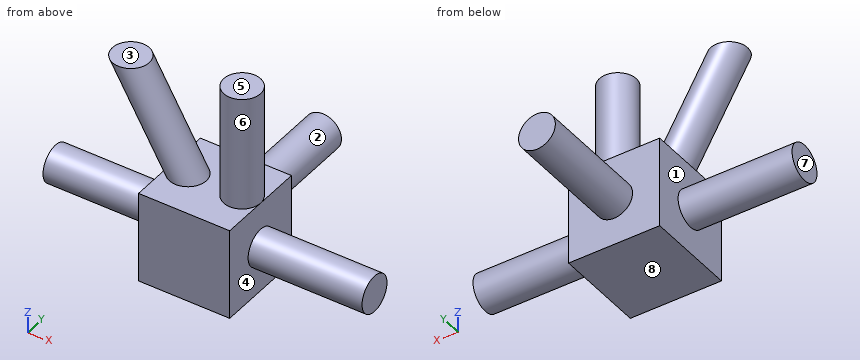
from build123d import *

# Parameters (mm, degrees)
F0_W      = 12
F0_H      = 12
F1_DEPTH  = 12
F2_R      = 2.425
F3_DEPTH  = 15
F4_R      = 2.425
F5_DEPTH  = 15
F6_R      = 2.425
F9_DEPTH  = 15
F10_R     = 2.425
F11_DEPTH = 15


with BuildPart() as f1:
    # F0 (on Top) → F1 (new body)
    with BuildSketch(Plane.XY):
        with Locations((-16.311498, 9.258204)):
            Rectangle(F0_W, F0_H)
    extrude(amount=F1_DEPTH)

    # F2 (on face) → F3 (join)
    with BuildSketch(Plane.YZ.offset(-10.311498)):
        with Locations((9.258204, 6)):
            Circle(F2_R)
    extrude(amount=F3_DEPTH)

    # F4 (on face) → F5 (join)
    with BuildSketch(Plane(origin=(-22.311498, 0, 0), x_dir=(0, -1, 0), z_dir=(-1, 0, 0))):
        with Locations((-9.258204, 6)):
            Circle(F4_R)
    extrude(amount=F5_DEPTH)

    # F8: sweep along a path in F7
    with BuildLine(Plane(origin=(0, 15.258204, 0), x_dir=(-1, 0, 0), z_dir=(0, 1, 0))) as f8_path:
        Line((19.886498, 12), (27.386498, 24.990381))
    # F6 (on face) → F8 (sweep)
    with BuildSketch(Plane.XY.offset(12)):
        with BuildLine():
            ThreePointArc((-22.311498, 9.258204), (-19.886498, 6.833204), (-17.461498, 9.258204))
            ThreePointArc((-17.461498, 9.258204), (-19.886498, 11.683204), (-22.311498, 9.258204))
        make_face()
    sweep(path=f8_path.line)

    # F6 (on face) → F9 (join)
    with BuildSketch(Plane.XY.offset(12)):
        with Locations((-12.736498, 9.258204)):
            Circle(F6_R)
    extrude(amount=F9_DEPTH)

    # F10 (on face) → F11 (join)
    with BuildSketch(Plane(origin=(0, 15.258204, 0), x_dir=(-1, 0, 0), z_dir=(0, 1, 0))):
        with Locations((16.311498, 6)):
            Circle(F10_R)
    extrude(amount=F11_DEPTH)


solid = f1.part
Can you work these out from the model? Positions are in its coordinate system, mm. Face numbers are marked on the shaded views. A direction names the side the tool comes from. Round coordinates to 2 decimals unless told otherwise and drop trailing zeros. Loops run counter-clockwise (first coordinate to the right, second up) from the corner with the lowest first, then second, coordinate; pieces in that order, holes last. Notation, with made-up numbers: (14.25, -22) - (54.25, -22) arc R22 ccw to (54.25, -9) - close; hole circle Ø11 at (38, -11). An arc over 180 degrees is marked (long way). Use CSV: the item, a comma, the result in double quotes. Start each with the question number.
1) We'd pull the mould along X, two halves only. Please class the marked faces 6, 7 and 8: released by +X, released by -X, zero draft, split by the parting line, or undercut.
2) If we section it at D-D on z = 9: Write out the boundary of the cut face in (x, y).
3) If we section it at B-B on y = 6.25: Write out the boundary of the cut face in (x, z), plus the area to 3 significant figures.
4) Please list where these lines run through material, in increasing order: probe 1 along X at (y, z) = (13, 5); probe 2 along Y at (x, z) = (-19, 5); probe 3 along X at (y, z) = (7.25, 19.5). Write a range as [from, to].
5) For the marked faces 1, 2, 3, 4 and 5, which set-ups out of +Z, -Z, +X, -X, +Y, -Y let a thin tool reach every point of the face, with its end or its side?
6) For pin 1 Ø1 at (x, y) = (-17, 16.5) entering from +Z; pin 2 Ø3 at (y, z) = (17.5, 7.5) entering from -X; pin 3 Ø4 at (y, z) = (11, 21.5) entering from -X; pin 4 Ø8 at (x, y) = (-1, 18) entering from +Z, each with a flat end and sliding along its axis, tell me the tip position at first contact or that it passes through.
7) If we section it at A-A on z = 6: Write out the boundary of the cut face in (x, y), plus the area to 3 significant figures.
Geometry results:
1,face 6,"undercut"
1,face 7,"released by -X"
1,face 8,"zero draft"
2,outline,"(-22.31, 3.26) - (-10.31, 3.26) - (-10.31, 15.26) - (-22.31, 15.26) - close"
3,outline,"(-22.31, 0) - (-10.31, 0) - (-10.31, 12) - (-22.31, 12) - close"
3,area,"144 mm2"
4,probe 1,"x = [-22.31, -10.31]"
4,probe 2,"y = [3.26, 15.26]"
4,probe 3,"x = [-25.58, -22.86], [-14.1, -11.38]"
5,face 1,"-X"
5,face 2,"+Y"
5,face 3,"+Z, -X, +Y, -Y"
5,face 4,"+X"
5,face 5,"+Z, +X, -X, +Y, -Y"
6,pin 1,"stops at z = 8.42"
6,pin 2,"stops at x = -18.74"
6,pin 3,"stops at x = -28.68"
6,pin 4,"passes through"
7,outline,"(-37.31, 6.83) - (-22.31, 6.83) - (-22.31, 3.26) - (-10.31, 3.26) - (-10.31, 6.83) - (4.69, 6.83) - (4.69, 11.68) - (-10.31, 11.68) - (-10.31, 15.26) - (-13.89, 15.26) - (-13.89, 30.26) - (-18.74, 30.26) - (-18.74, 15.26) - (-22.31, 15.26) - (-22.31, 11.68) - (-37.31, 11.68) - close"
7,area,"362 mm2"
